Could you check a few things on this model? Use its own coordinates, in mm. A direction names the side the tool comes from. Round coordinates to 2 decimals unless told otherwise and drop trailing zeros. Write each loop counter-clockwise with the first axis right and the second up, starting at its lowest first coordinate (ties: lowest second). Pieces come first, ordered by that corner, then holes. Notation, with made-up numbers: (-32.5, -18.75) -> (-4.5, -18.75) arc R16 cw to (-4.5, 5.25) -> close; hole circle Ø8 at (80, -9). An arc over 180 degrees is marked (long way). One line per question, with ' | ' between items. Start each with the question number.
1. For pin 1 Ø1.5 at (y, z) = (-1, 17.5) entering from +X; pin 2 Ø1.9 at (y, z) = (0, 121.51) entering from +X; pin 3 Ø2 at (x, z) = (1, 79.5) entering from +Y; pin 4 Ø1.5 at (y, z) = (-1.5, 27.5) entering from +X, each with a flat end and sliding along its axis, tell me the tip position at first contact or that it passes through.
2. If I drill on line 1 along Z through (x, y) = (-1, 0) (3 decimals); line 2 along Z through (x, y) = (0, 1) (3 decimals); line 3 along Z through (x, y) = (-3.25, 3) (3 decimals), over which ranges is the centre line in solid material (lowest first)? Write a range as [from, to].
3. For faces 1 (the flat face through (-4.445, 0, 131)), 2 (the cylindrical face through (-0.859, -3.868, 64.176)), which set-ups out of +Z, -Z, +X, -X, +Y, -Y let a thin tool reach every point of the face, with its end or its side?
4. Imagine slicing it at B-B, the plane x = 0. List the corners of the cut face in (y, z) for me (1 decimal), and give its area (3 significant figures).
5. Imagine slicing it at A-A, the plane y = 0. List the corners of the cut face in (x, z) for me (3 decimals), and give its area (3 significant figures).
6. Thinking about a two-plate mould opening in Z: for faces 3 (the cylindrical face through (0.055, -0.477, 123.028)), 4 (the flat face through (0, 0, 133.985)), 5 (the flat face through (0, 4.445, -1)), 6 (the cylindrical face through (0.054, -0.608, 10.128)), which applies, released by +Z, released by -Z, zero draft, split by the parting line, or undercut?
7. Imagine slicing it at C-C, the plane z = 83. List the corners of the cut face in (x, y) for me, and give its area (3 significant figures).
from build123d import *

# Parameters (mm, degrees)
SKETCH2_R           = 3.9624
BOSS_EXTRUDE1_DEPTH = 130.175
SKETCH3_W           = 16.328349939
SKETCH3_H           = 1.5875
SKETCH6_W           = 7.9248
SKETCH6_H           = 1.5875
SKETCH7_W           = 8.89
SKETCH7_H           = 8.89
BOSS_EXTRUDE2_DEPTH = 3.81
SKETCH8_W           = 8.89
SKETCH8_H           = 8.89
BOSS_EXTRUDE3_DEPTH = 3.81
FILLET1_R           = 1.27
FILLET2_R           = 1.27
FILLET3_R           = 1.27


with BuildPart() as part:
    # Sketch2 → Boss-Extrude1 (new body)
    with BuildSketch(Plane.XY):
        Circle(SKETCH2_R)
    extrude(amount=BOSS_EXTRUDE1_DEPTH)

    # Sketch3 → Cut-Revolve2 (revolve, cut)
    with BuildSketch(Plane(origin=(0, 0, 0), x_dir=(1, 0, 0), z_dir=(0, 1, 0)), mode=Mode.PRIVATE) as cut_revolve2_sk:
        with Locations((-0.379751444, -7.86765)):
            Rectangle(SKETCH3_W, SKETCH3_H)
    revolve(cut_revolve2_sk.sketch.rotate(Axis((7.784423526, 0, 8.6614), (-1, 0, 0)), 179.999999998), axis=Axis((7.784423526, 0, 8.6614), (-1, 0, 0)), mode=Mode.SUBTRACT)

    # Sketch6 → Cut-Revolve4 (revolve, cut)
    with BuildSketch(Plane(origin=(0, 0, 0), x_dir=(1, 0, 0), z_dir=(0, 1, 0))):
        with Locations((0, -122.30735)):
            Rectangle(SKETCH6_W, SKETCH6_H)
    revolve(axis=Axis((-3.9624, 0, 121.5136), (1, 0, 0)), mode=Mode.SUBTRACT)

    # Sketch7 → Boss-Extrude2 (add)
    with BuildSketch(Plane.XY.offset(130.175)):
        Rectangle(SKETCH7_W, SKETCH7_H)
    extrude(amount=BOSS_EXTRUDE2_DEPTH)

    # Sketch8 → Boss-Extrude3 (add)
    with BuildSketch(Plane(origin=(0, 0, 0), x_dir=(-1, 0, 0), z_dir=(0, 0, -1))):
        Rectangle(SKETCH8_W, SKETCH8_H)
    extrude(amount=BOSS_EXTRUDE3_DEPTH)

    # Fillet1
    fillet1_edges = [part.edges().sort_by_distance(p)[0] for p in [
        (0, 4.445, -3.81),
    ]]
    fillet(fillet1_edges, radius=FILLET1_R)

    # Fillet2
    fillet2_edges = [part.edges().sort_by_distance(p)[0] for p in [
        (-4.445, -4.445, -1.905),
        (4.445, -4.445, -1.905),
        (-4.445, -0.635, -3.81),
        (0, -4.445, -3.81),
        (4.445, -0.635, -3.81),
        (4.445, 4.445, -1.27),
        (4.445, 4.073025612, -3.438025612),
        (-4.445, 4.445, -1.27),
        (-4.445, 4.073025612, -3.438025612),
    ]]
    fillet(fillet2_edges, radius=FILLET2_R)

    # Fillet3
    fillet3_edges = [part.edges().sort_by_distance(p)[0] for p in [
        (4.445, -4.445, 132.08),
        (4.445, 4.445, 132.08),
        (-4.445, 4.445, 132.08),
        (-4.445, -4.445, 132.08),
        (4.445, 0, 133.985),
        (0, 4.445, 133.985),
        (-4.445, 0, 133.985),
        (0, -4.445, 133.985),
    ]]
    fillet(fillet3_edges, radius=FILLET3_R)


solid = part.part
Geometry results:
1) pin 1: stops at x = 3.95 | pin 2: passes through | pin 3: stops at y = 3.96 | pin 4: stops at x = 3.89
2) line 1: z = [-3.81, 7.074], [10.249, 119.926], [123.101, 133.985] | line 2: z = [-3.81, 7.428], [9.894, 120.281], [122.747, 133.985] | line 3: z = [-3.808, 0], [130.175, 133.983]
3) face 1: +Z, -Z, -X, +Y, -Y | face 2: none
4) outline: (-4.4, -2.5) arc R1.3 ccw to (-3.2, -3.8) -> (3.2, -3.8) arc R1.3 ccw to (4.4, -2.5) -> (4.4, 0) -> (4, 0) -> (4, 130.2) -> (4.4, 130.2) -> (4.4, 132.7) arc R1.3 ccw to (3.2, 134) -> (-3.2, 134) arc R1.3 ccw to (-4.4, 132.7) -> (-4.4, 130.2) -> (-4, 130.2) -> (-4, 0) -> (-4.4, 0) -> close; hole circle Ø3.2 at (0, 8.7); hole circle Ø3.2 at (0, 121.5) | area: 1,080 mm2
5) outline: (-4.445, -2.54) arc R1.27 ccw to (-3.175, -3.81) -> (3.175, -3.81) arc R1.27 ccw to (4.445, -2.54) -> (4.445, 0) -> (3.962, 0) -> (3.962, 7.074) -> (-3.962, 7.074) -> (-3.962, 0) -> (-4.445, 0) -> close; (-4.445, 130.175) -> (-3.962, 130.175) -> (-3.962, 123.101) -> (3.962, 123.101) -> (3.962, 130.175) -> (4.445, 130.175) -> (4.445, 132.715) arc R1.27 ccw to (3.175, 133.985) -> (-3.175, 133.985) arc R1.27 ccw to (-4.445, 132.715) -> close; (-3.962, 10.249) -> (3.962, 10.249) -> (3.962, 119.926) -> (-3.962, 119.926) -> close | area: 1,050 mm2
6) face 3: undercut | face 4: released by +Z | face 5: zero draft | face 6: undercut
7) outline: circle Ø7.92 at (0, 0) | area: 49.3 mm2
